Here's the drawing with two shaded views (mm, measured from the low corner). I have some questions. Round coordinates to 2 decimals unless told otherwise and drop trailing zeros. Loops run counter-clockwise (first coordinate to the right, second up) from the corner with the lowest first, then second, coordinate; pieces in that order, holes last.
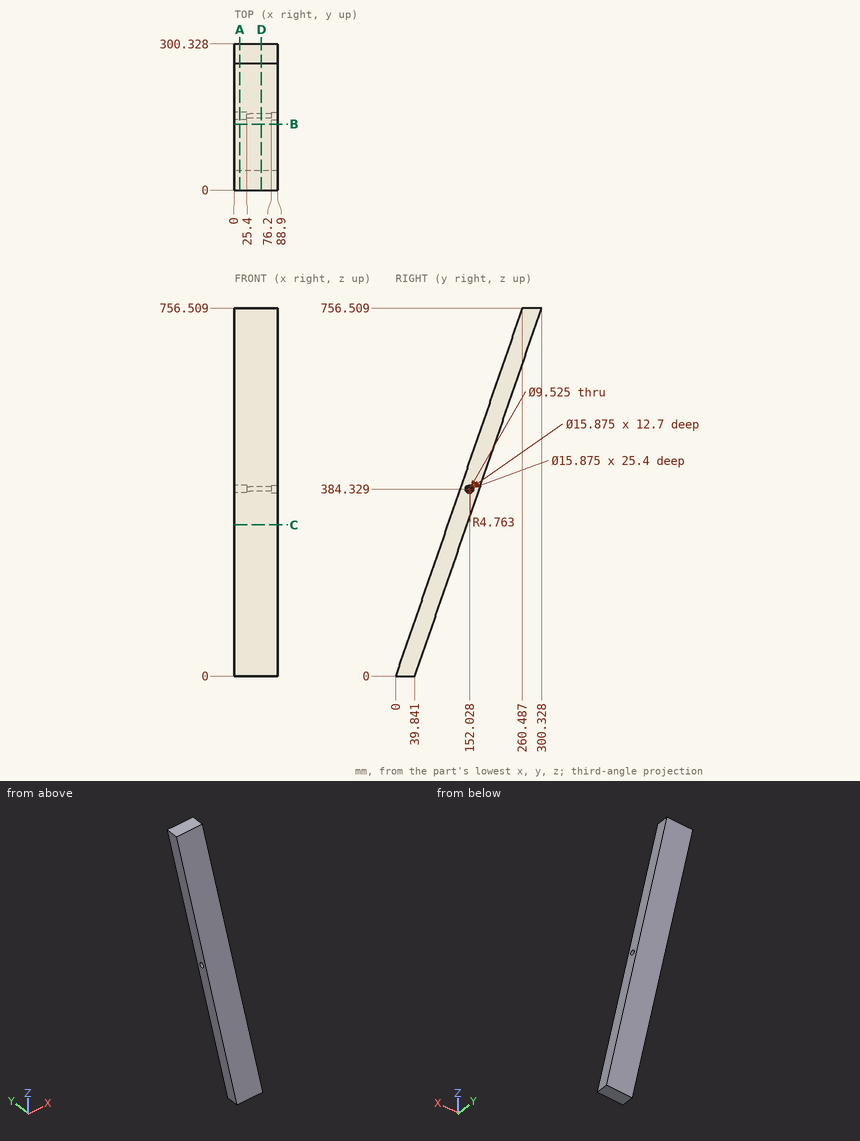
Item 1: If we section it at A-A, the plane x = 11.5: Please give me the cut outline in (y, z) (1 decimal), then the cut area to 3 significant figures.
Results list:
outline: (0, 0) - (39.8, 0) - (300.3, 756.5) - (260.5, 756.5) - close; hole circle Ø15.9 at (152, 384.3)
area: 29,900 mm2
Item 2: If we section it at D-D, the plane x = 55.5: Please give me the cut outline in (y, z) (1 decimal), then the cut area to 3 significant figures.
Results list:
outline: (0, 0) - (39.8, 0) - (300.3, 756.5) - (260.5, 756.5) - close; hole circle Ø9.5 at (152, 384.3)
area: 30,100 mm2
Item 3: If we section it at B-B, the plane y = 135.5: Please give me the cut outline in (x, z) (1 decimal), then the cut area to 3 significant figures.
Results list:
outline: (0, 277.8) - (88.9, 277.8) - (88.9, 393.5) - (0, 393.5) - close
area: 10,300 mm2
Item 4: If we section it at C-C, the plane z = 310.5: Please give me the cut outline in (x, y) (1 decimal).
Results list:
outline: (0, 106.9) - (88.9, 106.9) - (88.9, 146.8) - (0, 146.8) - close
Item 5: If I drill on line 1 along Y through (x, z) = (4, 384); line 2 along Y through (x, z) = (66, 155); line 3 along Y through (x, z) = (43, 473), over which ranges is the centre line in solid material (lowest first)?
Results list:
line 1: y = 132.22 to 144.1, 159.96 to 172.06
line 2: y = 53.37 to 93.21
line 3: y = 162.87 to 202.71
Item 6: Will these pins go through, and if not, where does the flat tip stop? pin 1 (1.5 mm diameter, centred on x = 16.5, z = 420, fed in from +Y); pin 2 (12.5 mm diameter, centred on y = 152.5, z = 384, fed in from -X); pin 3 (1.5 mm diameter, centred on x = 53, z = 251, fed in from -Y); pin 4 (7.5 mm diameter, centred on y = 152.03, z = 384.33, fed in from +X).
Results list:
pin 1: stops at y = 184.72
pin 2: stops at x = 25.4
pin 3: stops at y = 86.17
pin 4: passes through
